```python
from build123d import *

# Parameters (mm, degrees)
SKETCH_1_R               = 29.5
EXTRUDE_1_DEPTH          = 5
PATTERN_CIRCULAR_1_COUNT = 4
PATTERN_CIRCULAR_2_COUNT = 6


with BuildPart() as part:
    # 草图1 → 凸台-拉伸1 (new body)
    with BuildSketch(Plane(origin=(0, 0, 0), x_dir=(1, 0, 0), z_dir=(0, 1, 0))):
        with Locations(Location((0, 0, 0), (0, 0, 270))):
            Circle(SKETCH_1_R)
    extrude(amount=EXTRUDE_1_DEPTH)

    # 草图3 → M4 螺纹孔1 (revolve, cut)
    with BuildSketch(Plane(origin=(0, 5, -8), x_dir=(0, 0, 1), z_dir=(1, 0, 0))):
        Polygon((0, 0), (0, 11.091420021), (1.65, 10.1), (1.65, 0.375), (2.025, 0), align=None)
    hole_wizard_m4_1 = revolve(axis=Axis((0, 11.35, -8), (0, -1, 0)), mode=Mode.SUBTRACT)

    # 阵列(圆周)1: M4 螺纹孔1 ×4 about axis
    pattern_circular_1_axis = Axis((0, 0, 0.037874529), (0, 1, 0))
    for i in range(1, PATTERN_CIRCULAR_1_COUNT):
        add(hole_wizard_m4_1.rotate(pattern_circular_1_axis, i * 360 / PATTERN_CIRCULAR_1_COUNT), mode=Mode.SUBTRACT)

    # 草图5 → M4 螺纹孔2 (revolve, cut)
    with BuildSketch(Plane(origin=(0, 5, -17.25), x_dir=(0, 0, 1), z_dir=(1, 0, 0))):
        Polygon((0, 0), (0, 11.091420021), (1.65, 10.1), (1.65, 0.375), (2.025, 0), align=None)
    hole_wizard_m4_2 = revolve(axis=Axis((0, 11.35, -17.25), (0, -1, 0)), mode=Mode.SUBTRACT)

    # 阵列(圆周)2: M4 螺纹孔2 ×6 about axis
    pattern_circular_2_axis = Axis((0, 0, 0.082512271), (0, 1, 0))
    for i in range(1, PATTERN_CIRCULAR_2_COUNT):
        add(hole_wizard_m4_2.rotate(pattern_circular_2_axis, i * 360 / PATTERN_CIRCULAR_2_COUNT), mode=Mode.SUBTRACT)


solid = part.part
```
Geometry check sheet. Reference: the model listing, model coordinates, mm. Coordinates: 2 decimals unless noted, no trailing zeros. Write each loop counter-clockwise with the first axis right and the second up, starting at its lowest first coordinate (ties: lowest second). Pieces come first, ordered by that corner, then holes. Notation, with made-up numbers: M 53,-27 L 78,-27 A26 ccw 78,6 Z; hole C 54.25,-20.75 d2. An arc over 180 degrees is marked long. Use one line per item in the form item = value. Start each with the question number.
1) Go/stop test with a flat-tipped pin: pin 1 Ø2 at (x, y) = (14.5, 2.5) entering from +Z. Record where the tip stops, or that it passes through.
2) Section check B-B on y = 1.4. State how many separate pieces and enclosed holes the cut face has, and give its area (3 significant figures).
3) Thickness scan on probe 1 along Z at (x, y) = (13.5, 1.3); probe 2 along Z at (x, y) = (7, 4.3); probe 3 along Z at (x, y) = (16.5, 0.65). Record the ranges inside material, lowest first. Write a range as from..to.
4) Section check C-C on z = -17.25. Enter the section's corners in (x, y) (3 decimals).
5) Release check for a two-part mould opening along X. For faces 1 (the cylindrical face through (8.86, 2.46, 28.14)), 2 (the flat face through (0, 5, 0)), 3 (the cylindrical face through (-0.63, 2.34, 6.55)) record: pulls with the +X half, pulls with the -X half, needs draft (parallel to the pull), parting line crosses it, or undercut.
6) Section check D-D on z = 25. Enter the section's corners in (x, y).
7) Section check A-A on x = 0. Enter the section's corners in (y, z) (3 decimals), and give its area (3 significant figures).
Responses:
q1.pin_1 = 26.23
q2.separate_pieces = 1
q2.enclosed_holes = 10
q2.area = 2,650 mm2
q3.probe_1 = -26.23..-9.25, -7.92..8.08, 9.41..26.23
q3.probe_2 = -28.66..-1.24, 1.32..28.66
q3.probe_3 = -24.45..-9.29, -7.87..8.04, 9.46..24.45
q4.outline = M -23.931,0 L -1.65,0 L -1.65,4.625 L -2.025,5 L -23.931,5 Z; M 1.65,0 L 23.931,0 L 23.931,5 L 2.025,5 L 1.65,4.625 Z
q5.face_1 = parting line crosses it
q5.face_2 = needs draft
q5.face_3 = undercut
q6.outline = M -15.66,0 L 15.66,0 L 15.66,5 L -15.66,5 Z
q7.outline = M 0,-29.5 L 5,-29.5 L 5,-19.275 L 4.625,-18.9 L 0,-18.9 Z; M 0,-15.6 L 4.625,-15.6 L 5,-15.225 L 5,-10.025 L 4.625,-9.65 L 0,-9.65 Z; M 0,-6.35 L 4.625,-6.35 L 5,-5.975 L 5,6.051 L 4.625,6.426 L 0,6.426 Z; M 0,9.726 L 4.625,9.726 L 5,10.101 L 5,15.39 L 4.625,15.765 L 0,15.765 Z; M 0,19.065 L 4.625,19.065 L 5,19.44 L 5,29.5 L 0,29.5 Z
q7.area = 228 mm2
